Work out the finished part from the listing and answer in its coordinate system (mm). A direction names the side the tool comes from. Coordinates: 2 decimals unless noted, no trailing zeros. Order: outer loops, then holes, each group sorted by start corner. A loop starts at its lowest first (then second) coordinate and runs counter-clockwise, first axis right, second up.
```python
from build123d import *

# Parameters (mm, degrees)
F0_R     = 80
F0_R_2   = 2.5527
F0_R_3   = 39.9796
F0_R_4   = 2.5
F0_R_5   = 27.5209
F0_R_6   = 12.7
F1_DEPTH = 31.75
F2_DEPTH = 12.7
F3_DEPTH = 3.429


# Not quite as in the source:
# - a feature names something its author has since deleted; it is built from what else it names


with BuildPart() as f1:
    # F0 (on Front) → F1 (new body)
    with BuildSketch(Plane.XZ):
        Circle(F0_R)
        with Locations((-52.0854855022, -52.0854855022)):
            Circle(F0_R_2, mode=Mode.SUBTRACT)
        with Locations((-34.1249732601, -34.1249732601)):
            Circle(F0_R_2, mode=Mode.SUBTRACT)
        with Locations((0, -73.66)):
            Circle(F0_R_2, mode=Mode.SUBTRACT)
        with Locations((0, -48.26)):
            Circle(F0_R_2, mode=Mode.SUBTRACT)
        with Locations((52.0854855022, -52.0854855022)):
            Circle(F0_R_2, mode=Mode.SUBTRACT)
        with Locations((34.1249732601, -34.1249732601)):
            Circle(F0_R_2, mode=Mode.SUBTRACT)
        with Locations((-73.66, 0)):
            Circle(F0_R_2, mode=Mode.SUBTRACT)
        with Locations((-48.26, 0)):
            Circle(F0_R_2, mode=Mode.SUBTRACT)
        with Locations((-34.1249732601, 34.1249732601)):
            Circle(F0_R_2, mode=Mode.SUBTRACT)
        with Locations((-52.0854855022, 52.0854855022)):
            Circle(F0_R_2, mode=Mode.SUBTRACT)
        Circle(F0_R_3, mode=Mode.SUBTRACT)
        with Locations((34.1249732601, 34.1249732601)):
            Circle(F0_R_2, mode=Mode.SUBTRACT)
        with Locations((48.26, 0)):
            Circle(F0_R_2, mode=Mode.SUBTRACT)
        with Locations((73.66, 0)):
            Circle(F0_R_2, mode=Mode.SUBTRACT)
        with Locations((0, 48.26)):
            Circle(F0_R_2, mode=Mode.SUBTRACT)
        with Locations((0, 73.66)):
            Circle(F0_R_2, mode=Mode.SUBTRACT)
        with Locations((52.0854855022, 52.0854855022)):
            Circle(F0_R_2, mode=Mode.SUBTRACT)
        Circle(F0_R_3)
        with Locations((0, -32.8422)):
            Circle(F0_R_4, mode=Mode.SUBTRACT)
        with Locations((-32.8422, 0)):
            Circle(F0_R_4, mode=Mode.SUBTRACT)
        Circle(F0_R_5, mode=Mode.SUBTRACT)
        with Locations((32.8422, 0)):
            Circle(F0_R_4, mode=Mode.SUBTRACT)
        with Locations((0, 32.8422)):
            Circle(F0_R_4, mode=Mode.SUBTRACT)
        Circle(F0_R_5)
        with Locations((-16.1644610179, -16.1644610179)):
            Circle(F0_R_2, mode=Mode.SUBTRACT)
        with Locations((0, -22.86)):
            Circle(F0_R_2, mode=Mode.SUBTRACT)
        with Locations((16.1644610179, -16.1644610179)):
            Circle(F0_R_2, mode=Mode.SUBTRACT)
        with Locations((-22.86, 0)):
            Circle(F0_R_2, mode=Mode.SUBTRACT)
        with Locations((-16.1644610179, 16.1644610179)):
            Circle(F0_R_2, mode=Mode.SUBTRACT)
        Circle(F0_R_6, mode=Mode.SUBTRACT)
        with Locations((16.1644610179, 16.1644610179)):
            Circle(F0_R_2, mode=Mode.SUBTRACT)
        with Locations((22.86, 0)):
            Circle(F0_R_2, mode=Mode.SUBTRACT)
        with Locations((0, 22.86)):
            Circle(F0_R_2, mode=Mode.SUBTRACT)
        with Locations((0, 32.8422)):
            Circle(F0_R_4)
        with Locations((0, -32.8422)):
            Circle(F0_R_4)
        with Locations((32.8422, 0)):
            Circle(F0_R_4)
        with Locations((-32.8422, 0)):
            Circle(F0_R_4)
    extrude(amount=-F1_DEPTH)

    # F0 (on Front) → F2 (cut)
    with BuildSketch(Plane.XZ):
        with Locations((0, 32.8422)):
            Circle(F0_R_4)
        with Locations((32.8422, 0)):
            Circle(F0_R_4)
        with Locations((0, -32.8422)):
            Circle(F0_R_4)
        with Locations((-32.8422, 0)):
            Circle(F0_R_4)
    extrude(amount=-F2_DEPTH, mode=Mode.SUBTRACT)

    # F0 (on Front) → F3 (cut)
    with BuildSketch(Plane.XZ):
        Circle(F0_R_5)
        with Locations((-16.1644610179, -16.1644610179)):
            Circle(F0_R_2, mode=Mode.SUBTRACT)
        with Locations((0, -22.86)):
            Circle(F0_R_2, mode=Mode.SUBTRACT)
        with Locations((16.1644610179, -16.1644610179)):
            Circle(F0_R_2, mode=Mode.SUBTRACT)
        with Locations((-22.86, 0)):
            Circle(F0_R_2, mode=Mode.SUBTRACT)
        with Locations((-16.1644610179, 16.1644610179)):
            Circle(F0_R_2, mode=Mode.SUBTRACT)
        Circle(F0_R_6, mode=Mode.SUBTRACT)
        with Locations((16.1644610179, 16.1644610179)):
            Circle(F0_R_2, mode=Mode.SUBTRACT)
        with Locations((22.86, 0)):
            Circle(F0_R_2, mode=Mode.SUBTRACT)
        with Locations((0, 22.86)):
            Circle(F0_R_2, mode=Mode.SUBTRACT)
    extrude(amount=-F3_DEPTH, mode=Mode.SUBTRACT)


solid = f1.part
```
1. Flat-ended cylindrical pins translate along their axes: pin 1 (6 mm diameter, centred on y = 4.5, z = 45, fed in from -X); pin 2 (10 mm diameter, centred on y = 19, z = 63.5, fed in from -X); pin 3 (4 mm diameter, centred on y = 12.5, z = 10, fed in from -X); pin 4 (8 mm diameter, centred on x = 0, z = 48.26, fed in from -Y). Find the tip coordinate at first contact, or state that the pin passes through.
2. Consider probe 1 along X at (y, z) = (9.5, -33); probe 2 along Z at (x, y) = (54, 3); probe 3 along X at (y, z) = (26, -34.5). Determine where each line is inside the solid, lowest interval first.
3. The part is cut by section B-B (z = -73.66). Determine the outline of the cut face in (x, y), plus the area to 3 significant figures.
4. The part is cut by section A-A (x = 33.5). Determine the outline of the cut face in (y, z).
5. The part is cut by section C-C (y = 9.5). Count the separate pieces of the cut face and the enclosed holes in it, plus the area to 3 significant figures.
6. The part is cut by section D-D (x = -73.66). Determine the outline of the cut face in (y, z), plus the area to 3 significant figures.
7. The mould has two halves that part along X. Classify faces 1 (the flat face through (-1, 31.75, -17)), 2 (the cylindrical face through (-18.19, 17.39, 14.61)), 3 (the cylindrical face through (45.71, 15.65, 0.11)): released by +X, released by -X, zero draft, split by the parting line, or undercut.
8. For faces 4 (the cylindrical face through (-0.542, 6.261, -35.283)), 5 (the cylindrical face through (-0.33, 15.65, 76.19)), determine the directions among +Z, -Z, +X, -X, +Y, -Y from which every point of the face is accessible in a straight line to the end or side of a thin tool.
Worked out:
1. pin 1: stops at x = -68.09
1. pin 2: stops at x = -54.57
1. pin 3: stops at x = -79.6
1. pin 4: stops at y = 0
2. probe 1: x = -72.88 to -36.42, -31.83 to -2.5, 2.5 to 31.83, 36.42 to 72.88
2. probe 2: z = -59.03 to -53.77, -50.4 to 50.4, 53.77 to 59.03
2. probe 3: x = -72.18 to -36.65, -31.6 to 31.6, 36.65 to 72.18
3. outline: (-31.21, 0) - (-2.55, 0) - (-2.55, 31.75) - (-31.21, 31.75) - close; (2.55, 0) - (31.21, 0) - (31.21, 31.75) - (2.55, 31.75) - close
3. area: 1,820 mm2
4. outline: (0, -72.65) - (31.75, -72.65) - (31.75, -36.6) - (0, -36.6) - close; (0, -31.65) - (31.75, -31.65) - (31.75, 31.65) - (0, 31.65) - (0, 2.41) - (12.7, 2.41) - (12.7, -2.41) - (0, -2.41) - close; (0, 36.6) - (31.75, 36.6) - (31.75, 72.65) - (0, 72.65) - close
5. separate pieces: 1
5. enclosed holes: 29
5. area: 19,000 mm2
6. outline: (0, -31.21) - (31.75, -31.21) - (31.75, -2.55) - (0, -2.55) - close; (0, 2.55) - (31.75, 2.55) - (31.75, 31.21) - (0, 31.21) - close
6. area: 1,820 mm2
7. face 1: zero draft
7. face 2: undercut
7. face 3: undercut
8. face 4: -Y
8. face 5: +Y, -Y
